Design review of the part shown in the three views and the two pictorial views. Dimensions are in mm from the part's minimum x, y and z. A direction names the side the tool comes from. Round coordinates to 2 decimals unless told otherwise and drop trailing zeros. Loops run counter-clockwise (first coordinate to the right, second up) from the corner with the lowest first, then second, coordinate; pieces in that order, holes last.
1) Take a section at B-B (y = 124). State the section outline as (x, z) points.
2) Take a section at C-C (x = 17). State the section outline as (y, z) points, then the cut area to 3 significant figures.
3) Take a section at A-A (z = 15.5). State the section outline as (x, y) points, then the cut area to 3 significant figures.
4) Insertion check: pin 1 (5 mm diameter, centred on x = 13.5, y = 31.5, fed in from +Z); pin 2 (2 mm diameter, centred on y = 170, z = 2.5, fed in from +X); pin 3 (1.5 mm diameter, centred on y = 72, z = 7, fed in from +X); pin 4 (2 mm diameter, centred on y = 235, z = 9.5, fed in from +X). Each pin has a flat end and moves straight along its axis. Give the tip position at first contact, or say it passes through.
5) Tool access review of the marked faces 1 and 2: name each direction out of +Z, -Z, +X, -X, +Y, -Y from which nothing blocks a thin tool from reaching the whole face with its end or side.
6) Wall thickness on L1, parallel to Y at x = 3.5, z = 8.5; L2, parallel to Y at x = 6, z = 8.75; L3, parallel to Y at x = 17.5, z = 7: over which ranges is each line inside the solid? List them lowest first.
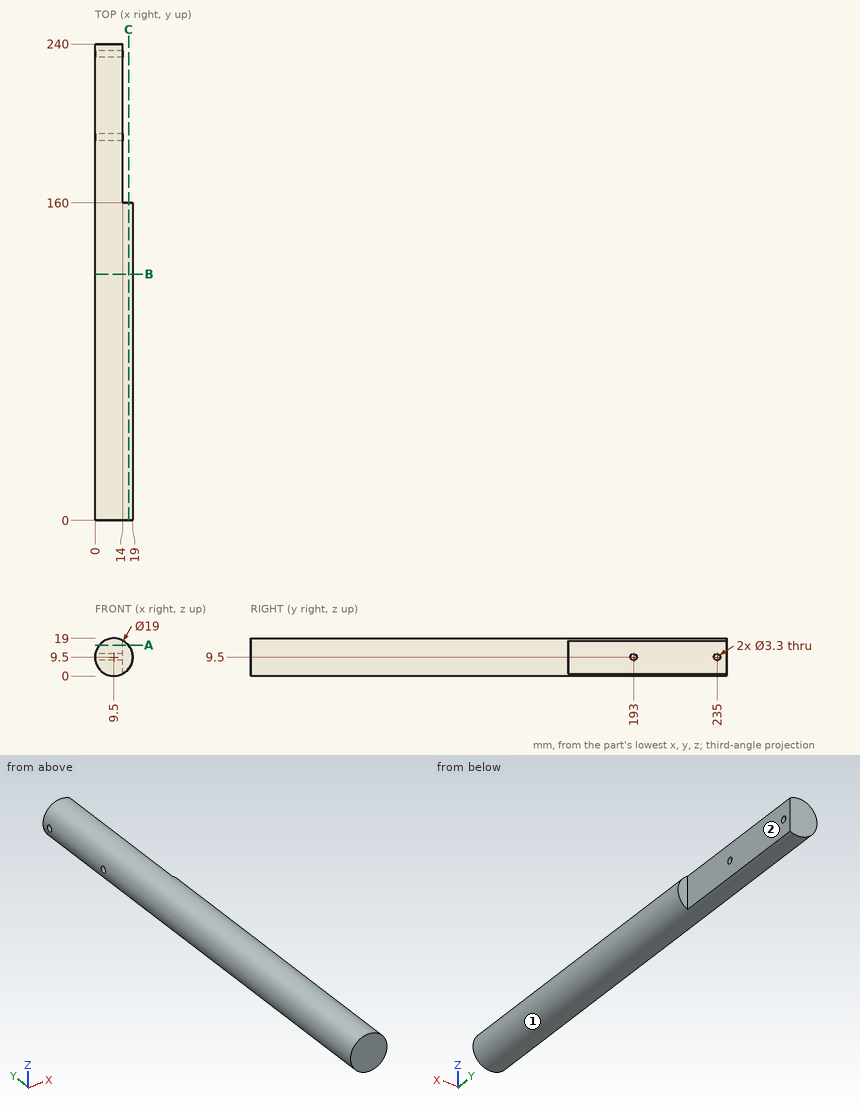
Response:
1. outline: circle Ø19 at (9.5, 9.5)
2. outline: (0, 3.67) - (160, 3.67) - (160, 15.33) - (0, 15.33) - close
2. area: 1,870 mm2
3. outline: (2.13, 0) - (16.87, 0) - (16.87, 160) - (14, 160) - (14, 240) - (2.13, 240) - close
3. area: 3,310 mm2
4. pin 1: stops at z = 18.88
4. pin 2: stops at x = 14
4. pin 3: stops at x = 18.84
4. pin 4: passes through
5. face 1: +Y, -Y
5. face 2: +Z, -Z, +X, +Y
6. L1: y = 0 to 191.69, 194.31 to 233.69, 236.31 to 240
6. L2: y = 0 to 191.53, 194.47 to 233.53, 236.47 to 240
6. L3: y = 0 to 160
